from build123d import *

# Parameters (mm, degrees)
BASE_FLANGE1_DEPTH   = 16.5
SKETCH6_R            = 4
CUT_EXTRUDE1_DEPTH   = 58.247270677
M5_CLEARANCE_HOLE1_D = 5.8
FILLET1_R            = 10


# Sheet-metal steps are written as plain solids
with BuildPart() as part:
    # Sketch1 → Base-Flange1 (new, symmetric)
    with BuildSketch(Plane.XY):
        with BuildLine():
            Line((43, 15.5), (1.5, 15.5))
            ThreePointArc((1.5, 15.5), (0.439339828, 15.060660172), (0, 14))
            Line((0, 14), (0, -14))
            ThreePointArc((0, -14), (0.439339828, -15.060660172), (1.5, -15.5))
            Line((1.5, -15.5), (43, -15.5))
            Line((43, -15.5), (43, -17))
            Line((43, -17), (1.5, -17))
            ThreePointArc((1.5, -17), (-0.621320344, -16.121320344), (-1.5, -14))
            Line((-1.5, -14), (-1.5, 14))
            ThreePointArc((-1.5, 14), (-0.621320344, 16.121320344), (1.5, 17))
            Line((1.5, 17), (43, 17))
            Line((43, 17), (43, 15.5))
        make_face()
    extrude(amount=BASE_FLANGE1_DEPTH, both=True)

    # Sketch6 → Cut-Extrude1 (cut, through all)
    with BuildSketch(Plane(origin=(0, 17, 0), x_dir=(1, 0, 0), z_dir=(0, 1, 0))):
        with Locations(Location((26.5, 0, 0), (0, 0, 270))):
            Circle(SKETCH6_R)
    extrude(amount=-CUT_EXTRUDE1_DEPTH, mode=Mode.SUBTRACT)

    # M5 Clearance Hole1 (through all)
    with Locations(Plane.ZY.offset(1.5)):
        with Locations((0, 0)):
            Hole(M5_CLEARANCE_HOLE1_D / 2)

    # Fillet1
    fillet1_edges = [part.edges().sort_by_distance(p)[0] for p in [
        (43, 16.25, -16.5),
        (43, -16.25, -16.5),
        (43, 16.25, 16.5),
        (43, -16.25, 16.5),
    ]]
    fillet(fillet1_edges, radius=FILLET1_R)


solid = part.part
Design review of the part built by this model. Coordinates are the model's own, in mm. A direction names the side the tool comes from. Give positions to 0.01 mm unless a question says otherwise; leave off trailing zeros. Write each loop counter-clockwise with the first axis right and the second up, starting at its lowest first coordinate (ties: lowest second). Pieces come first, ordered by that corner, then holes. Notation, with made-up numbers: M 12,32.5 L 46,32.5 A21 ccw 46,55.5 Z; hole C 76,52 d9. An arc over 180 degrees is marked long. Answer as a JSON object with one key per item and string values. Group by question number.
1) Tool access review of faces 5 (the face through (23, 15.5, 4)), 6 (the face through (-0.7, 0.1, 2.9)): name each direction out of +Z, -Z, +X, -X, +Y, -Y from which nothing blocks a thin tool from reaching the whole face with its end or side.
2) We need section D-D (x = 26.5). Give the boundary of the cut face in (y, z), and give its area (3 significant figures).
3) We need section C-C (z = 0). Give the boundary of the cut face in (x, y).
4) Mouldability with a two-part tool opening along Z and no side actions: class faces 1 (the face through (39.99, -16.26, 13.65)), 2 (the face through (30.466, 16.26, -0.521)), 3 (the face through (0, 3.3, 0.2)), 4 (the face through (30.466, -16.24, -0.521)) as released by +Z, released by -Z, zero draft, split by the parting line, or undercut.
5) We need section B-B (y = 0). Give the boundary of the cut face in (x, z), and give its area (3 significant figures).
6) For line 1 along Y through (x, z) = (5.5, -12.5); line 2 along Z through (x, y) = (26, 16); line 3 along X through (y, z) = (-1.5, -10), list the stretches that pass through material, from the lowest coordinate up.
7) Clearance check with flat-ended pins moving along their axes: pin 1 Ø6.5 at (x, z) = (26.5, 0) entering from +Y; pin 2 Ø2 at (y, z) = (2.5, -7.5) entering from +X. State where each tip first meets the part, or that it passes through.
8) We need section A-A (x = 3.5). Give the boundary of the cut face in (y, z), and give its area (3 significant figures).
Answer key:
{
 "1": {"face 5": "+Z, -Z, +X", "face 6": "+X, -X"},
 "2": {"outline": "M -17,-16.5 L -15.5,-16.5 L -15.5,-4 L -17,-4 Z; M -17,4 L -15.5,4 L -15.5,16.5 L -17,16.5 Z; M 15.5,-16.5 L 17,-16.5 L 17,-4 L 15.5,-4 Z; M 15.5,4 L 17,4 L 17,16.5 L 15.5,16.5 Z", "area": "75.0 mm²"},
 "3": {"outline": "M -1.5,-14 A3 ccw 1.5,-17 L 22.5,-17 L 22.5,-15.5 L 1.5,-15.5 A1.5 cw 0,-14 L 0,-2.9 L -1.5,-2.9 Z; M -1.5,2.9 L 0,2.9 L 0,14 A1.5 cw 1.5,15.5 L 22.5,15.5 L 22.5,17 L 1.5,17 A3 ccw -1.5,14 Z; M 30.5,-17 L 43,-17 L 43,-15.5 L 30.5,-15.5 Z; M 30.5,15.5 L 43,15.5 L 43,17 L 30.5,17 Z"},
 "4": {"face 1": "released by +Z", "face 2": "undercut", "face 3": "zero draft", "face 4": "undercut"},
 "5": {"outline": "M -1.5,-16.5 L 0,-16.5 L 0,-2.9 L -1.5,-2.9 Z; M -1.5,2.9 L 0,2.9 L 0,16.5 L -1.5,16.5 Z", "area": "40.8 mm²"},
 "6": {"line 1": "y = -17 to -15.5, 15.5 to 17", "line 2": "z = -16.5 to -3.97, 3.97 to 16.5", "line 3": "x = -1.5 to 0"},
 "7": {"pin 1": "passes through", "pin 2": "stops at x = 0"},
 "8": {"outline": "M -17,-16.5 L -15.5,-16.5 L -15.5,16.5 L -17,16.5 Z; M 15.5,-16.5 L 17,-16.5 L 17,16.5 L 15.5,16.5 Z", "area": "99.0 mm²"}
}
